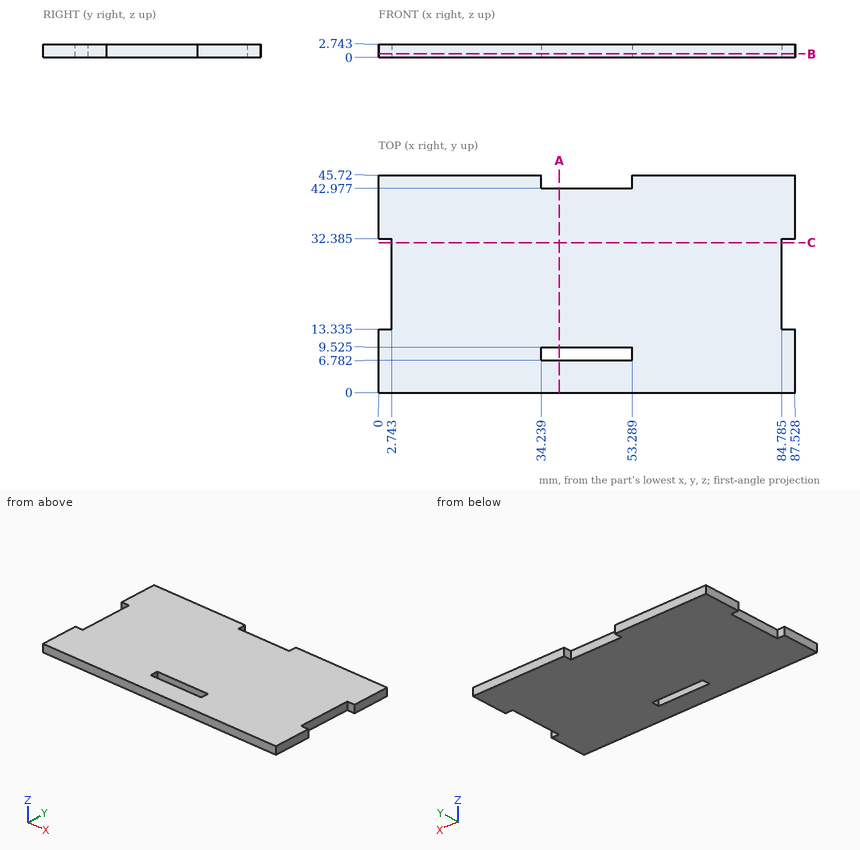
Geometry: see drawing. Coordinates: mm, zero at the bounding-box minimum. Coordinates: 2 decimals unless noted, no trailing zeros. Loops run counter-clockwise (first coordinate to the right, second up) from the corner with the lowest first, then second, coordinate; pieces in that order, holes last. Notation, with made-up numbers: (73.25, -19) -> (109.25, -19) arc R20 cw to (109.25, 1) -> close; hole circle Ø3 at (60, -27.5). An arc over 180 degrees is marked (long way). Use a Markdown table: item, result.
1) Cut plane B-B (z = 0.65). Return the cut outline in (x, y) (1 decimal), then the cut area to 3 significant figures.
Results found:
| item | result |
|---|---|
| outline | (0, 0) -> (87.5, 0) -> (87.5, 13.3) -> (84.8, 13.3) -> (84.8, 32.4) -> (87.5, 32.4) -> (87.5, 45.7) -> (53.3, 45.7) -> (53.3, 43) -> (34.2, 43) -> (34.2, 45.7) -> (0, 45.7) -> (0, 32.4) -> (2.7, 32.4) -> (2.7, 13.3) -> (0, 13.3) -> close; hole (34.2, 6.8) -> (53.3, 6.8) -> (53.3, 9.5) -> (34.2, 9.5) -> close |
| area | 3,790 mm2 |
2) Contact query for flat-ended pins moving along their axis: pin 1 (1 mm diameter, centred on y = 18.5, z = 1, fed in from -X); pin 2 (0.8 mm diameter, centred on x = 47, z = 1.5, fed in from +Y). Output: stop coordinate, or through.
Results found:
| item | result |
|---|---|
| pin 1 | stops at x = 2.74 |
| pin 2 | stops at y = 42.98 |
3) Material intervals for line 1 along Y through (x, z) = (36, 1.05) (1 decimal); line 2 along X through (y, z) = (14.5, 2.45) (1 decimal), sorted ascending. Write a range as from..to.
Results found:
| item | result |
|---|---|
| line 1 | y = 0..6.8, 9.5..43 |
| line 2 | x = 2.7..84.8 |
4) Cut plane C-C (y = 31.5). Return the cut outline in (x, z) (1 decimal).
Results found:
| item | result |
|---|---|
| outline | (2.7, 0) -> (84.8, 0) -> (84.8, 2.7) -> (2.7, 2.7) -> close |
5) Cut plane A-A (x = 38). Return the cut outline in (y, z) (1 decimal).
Results found:
| item | result |
|---|---|
| outline | (0, 0) -> (6.8, 0) -> (6.8, 2.7) -> (0, 2.7) -> close; (9.5, 0) -> (43, 0) -> (43, 2.7) -> (9.5, 2.7) -> close |
